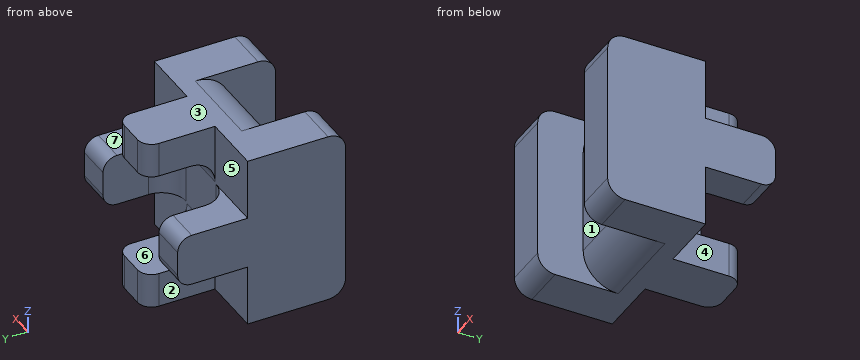
from build123d import *

# Parameters (mm, degrees)
BOX_W        = 10
BOX_H        = 3
BOX_DEPTH    = 10
SKETCH_W     = 3
SKETCH_H     = 2
SKETCH_W_2   = 2
SKETCH_H_2   = 3
PAD_DEPTH    = 4
SKETCH001_W  = 2.5
SKETCH001_H  = 10
PAD001_DEPTH = 2.6
FILLET_R     = 2
FILLET001_R  = 0.8
FILLET002_R  = 1
FILLET003_R  = 1.4


with BuildPart() as part:
    # Box → Box (new body)
    with BuildSketch(Plane(origin=(-5, 0, -5), x_dir=(1, 0, 0), z_dir=(0, 0, 1))):
        with Locations((5, 1.5)):
            Rectangle(BOX_W, BOX_H)
    extrude(amount=BOX_DEPTH)

    # Sketch → Pad (new body)
    with BuildSketch(Plane(origin=(-5, 3, -5), x_dir=(-1, 0, 0), z_dir=(0, 1, 0))):
        with Locations((-5, 9)):
            Rectangle(SKETCH_W, SKETCH_H)
        with Locations((-9, 5)):
            Rectangle(SKETCH_W_2, SKETCH_H_2)
        with Locations((-1, 5)):
            Rectangle(SKETCH_W_2, SKETCH_H_2)
        with Locations((-5, 1)):
            Rectangle(SKETCH_W, SKETCH_H)
    extrude(amount=PAD_DEPTH)

    # Sketch001 → Pad001 (new body)
    with BuildSketch(Plane(origin=(-5, 0, -5), x_dir=(1, 0, 0), z_dir=(0, -1, 0))):
        with Locations((1.25, 5)):
            Rectangle(SKETCH001_W, SKETCH001_H)
        with Locations((8.75, 5)):
            Rectangle(SKETCH001_W, SKETCH001_H)
    extrude(amount=PAD001_DEPTH)

    # Fillet
    fillet_edges = [part.edges().sort_by_distance(p)[0] for p in [
        (0, 0, -5),
        (0, 0, 5),
    ]]
    fillet(fillet_edges, radius=FILLET_R)

    # Fillet001
    fillet001_edges = [part.edges().sort_by_distance(p)[0] for p in [
        (4, 7, -1.5),
        (4, 7, 1.5),
        (1.5, 7, 4),
        (-1.5, 7, 4),
        (-4, 7, 1.5),
        (-4, 7, -1.5),
        (-1.5, 7, -4),
        (1.5, 7, -4),
    ]]
    fillet(fillet001_edges, radius=FILLET001_R)

    # Fillet002
    fillet002_edges = [part.edges().sort_by_distance(p)[0] for p in [
        (-3.75, -2.6, -5),
        (3.75, -2.6, -5),
        (3.75, -2.6, 5),
        (-3.75, -2.6, 5),
    ]]
    fillet(fillet002_edges, radius=FILLET002_R)

    # Fillet003
    fillet003_edges = [part.edges().sort_by_distance(p)[0] for p in [
        (0, 3, -3),
        (-3, 3, 0),
        (3, 3, 0),
        (0, 3, 3),
    ]]
    fillet(fillet003_edges, radius=FILLET003_R)


solid = part.part
The model under review builds one solid part; all positions refer to its coordinate system, in mm. Face numbers are marked on the shaded views. A direction names the side the tool comes from. Coordinates: 2 decimals unless noted, no trailing zeros. Loops run counter-clockwise (first coordinate to the right, second up) from the corner with the lowest first, then second, coordinate; pieces in that order, holes last. Notation, with made-up numbers: M 55.25,-36.75 L 93.25,-36.75 A26 cw 93.25,-15.75 Z; hole C 12.25,31.25 d6. An arc over 180 degrees is marked long. Put each result on its own line as item: value. Start each with the question number.
Q1. Clearance check with flat-ended pins moving along their axes: pin 1 (1.6 mm diameter, centred on x = 4, y = 4.5, fed in from +Z); pin 2 (1.5 mm diameter, centred on x = 1, z = 0.5, fed in from -Y); pin 3 (1 mm diameter, centred on x = 3, y = 4, fed in from -Z). State where each tip first meets the part, or that it passes through.
Q2. Add section A-A (x = -0.5). Write out the cut boundary in (y, z).
Q3. Add section B-B (z = -2). Write out the cut boundary in (x, y), and give its area (3 significant figures).
Q4. Add section C-C (y = 3.75). Write out the cut boundary in (x, z).
Q5. Add section D-D (x = 2). Write out the cut boundary in (y, z), and give its area (3 significant figures).
Q6. Wall thickness on line 1 (X direction, y = -0.25, z = -4.5); line 2 (X direction, y = 6.75, z = -1.25); line 3 (Y direction, x = -3.75, z = -3.5): over which ranges is each line inside the solid? List them lowest first.
Q7. The part is to be moulded in two halves that separate along X. For the marked faces 1, 2 and 3, say which applies: +X half, -X half, draft (parallel to the pull), parting line (faces both ways), or undercut.
Q8. For the marked faces 4, 5, 6 and 7, list the 3-axis set-ups (+Z, -Z, +X, -X, +Y, -Y) from which the entire face can be reached by the end or side of a thin tool; tool diameter is ignored.
Answers:
1. pin 1: stops at z = 1.5
1. pin 2: stops at y = 0
1. pin 3: stops at z = -1.5
2. outline: M 0,-3 A2 ccw 2,-5 L 7,-5 L 7,-3 L 4.4,-3 A1.4 cw 3,-1.6 L 3,1.6 A1.4 cw 4.4,3 L 7,3 L 7,5 L 2,5 A2 ccw 0,3 Z
3. outline: M -5,-2.6 L -2.5,-2.6 L -2.5,0 L 2.5,0 L 2.5,-2.6 L 5,-2.6 L 5,3 L 1.5,3 L 1.5,3.06 L -1.5,3.06 L -1.5,3 L -5,3 Z
3. area: 43.2 mm^2
4. outline: M -5,-1.5 L -2.84,-1.5 L -2.84,1.5 L -5,1.5 Z; M -1.5,-5 L 1.5,-5 L 1.5,-2.84 L -1.5,-2.84 Z; M -1.5,2.84 L 1.5,2.84 L 1.5,5 L -1.5,5 Z; M 2.84,-1.5 L 5,-1.5 L 5,1.5 L 2.84,1.5 Z
5. outline: M 0,-3 A2 ccw 2,-5 L 3,-5 L 3,-1.5 L 3.06,-1.5 L 3.06,1.5 L 3,1.5 L 3,5 L 2,5 A2 ccw 0,3 Z
5. area: 28.5 mm^2
6. line 1: x = -5 to -2.5, 2.5 to 5
6. line 2: x = -5 to -3, 3 to 5
6. line 3: y = -2.6 to 3
7. face 1: undercut
7. face 2: -X half
7. face 3: draft
8. face 4: +Z, -Z, +X, +Y
8. face 5: +Y
8. face 6: +X, -X, +Y
8. face 7: +Z, +X, -X, +Y
